The model under review builds one solid part; all positions refer to its coordinate system, in mm. A direction names the side the tool comes from. Coordinates: 2 decimals unless noted, no trailing zeros. Write each loop counter-clockwise with the first axis right and the second up, starting at its lowest first coordinate (ties: lowest second). Pieces come first, ordered by that corner, then holes. Notation, with made-up numbers: (50.25, 71.5) - (81.25, 71.5) arc R19 cw to (81.25, 87.5) - close; hole circle Ø7 at (-18.5, 46.25). An arc over 180 degrees is marked (long way). Put each result on its own line as item: value.
from build123d import *

# Parameters (mm, degrees)
SZKIC1_R                    = 1.5
DODANIE_WYCI_GNI_CIE1_DEPTH = 2
SZKIC2_W                    = 3
SZKIC2_H                    = 6
DODANIE_WYCI_GNI_CIE2_DEPTH = 10
SZKIC3_R                    = 1.5
WYTNIJ_WYCI_GNI_CIE1_DEPTH  = 3
SFAZOWANIE1_SIZE            = 1
SFAZOWANIE2_SIZE            = 1


with BuildPart() as part:
    # Szkic1 → Dodanie-wyciągnięcie1 (new body)
    with BuildSketch(Plane.XY):
        with BuildLine():
            Line((-6.716548808, 4.5), (7.283451192, 4.5))
            Line((7.283451192, 4.5), (7.283451192, 10.768070335))
            ThreePointArc((7.283451192, 10.768070335), (0.336426694, 12.995646082), (-6.716548808, 11.130497388))
            Line((-6.716548808, 11.130497388), (-6.716548808, 4.5))
        make_face()
        with Locations((0.283451192, 10.49617337)):
            Circle(SZKIC1_R, mode=Mode.SUBTRACT)
    extrude(amount=DODANIE_WYCI_GNI_CIE1_DEPTH)

    # Szkic2 → Dodanie-wyciągnięcie2 (add)
    with BuildSketch(Plane.XY.offset(2)):
        with Locations((5.783451192, 7.5)):
            Rectangle(SZKIC2_W, SZKIC2_H)
    extrude(amount=DODANIE_WYCI_GNI_CIE2_DEPTH)

    # Szkic3 → Wytnij-wyciągnięcie1 (cut)
    with BuildSketch(Plane.ZY.offset(-4.283451192)):
        with Locations((9, 7.579153313)):
            Circle(SZKIC3_R)
    extrude(amount=-WYTNIJ_WYCI_GNI_CIE1_DEPTH, mode=Mode.SUBTRACT)

    # Sfazowanie1
    sfazowanie1_edges = [part.edges().sort_by_distance(p)[0] for p in [
        (4.283451192, 7.5, 2),
    ]]
    chamfer(sfazowanie1_edges, length=SFAZOWANIE1_SIZE)

    # Sfazowanie2
    sfazowanie2_edges = [part.edges().sort_by_distance(p)[0] for p in [
        (5.283451192, 10.5, 2),
    ]]
    chamfer(sfazowanie2_edges, length=SFAZOWANIE2_SIZE)


solid = part.part
1. Consider section D-D on z = 5.5. State the section outline as (x, y) points.
Determined:
outline: (4.28, 4.5) - (7.28, 4.5) - (7.28, 10.5) - (4.28, 10.5) - close
2. To check wall thickness, follow probe 1 along X at (y, z) = (10.5, 0.5); probe 2 along X at (y, z) = (10.25, 6.25); probe 3 along Z at (x, y) = (-4.5, 10.25). State the ranges of each line that lie inside material, in increasing order.
Determined:
probe 1: x = -6.72 to -1.22, 1.78 to 7.28
probe 2: x = 4.28 to 7.28
probe 3: z = 0 to 2
3. Consider section B-B on y = 9.5. State the section outline as (x, z) points, plus the area to 3 significant figures.
Determined:
outline: (-6.72, 0) - (-0.84, 0) - (-0.84, 2) - (-6.72, 2) - close; (1.4, 0) - (7.28, 0) - (7.28, 12) - (4.28, 12) - (4.28, 3) - (3.28, 2) - (1.4, 2) - close
area: 54.0 mm^2
4. Consider section A-A on z = 9. State the section outline as (x, y) points.
Determined:
outline: (4.28, 4.5) - (7.28, 4.5) - (7.28, 6.08) - (4.28, 6.08) - close; (4.28, 9.08) - (7.28, 9.08) - (7.28, 10.5) - (4.28, 10.5) - close
5. For pin 1 Ø2 at (x, z) = (-5, 2) entering from +Y; pin 2 Ø4.5 at (x, y) = (0.5, 7) entering from +Z; pin 3 Ø0.9 at (x, z) = (5, 8.5) entering from +Y, all flat-tipped, find the tip position at first contact; note any pin that passes through.
Determined:
pin 1: stops at y = 12.37
pin 2: stops at z = 2
pin 3: stops at y = 10.5
6. Machinability: for faces 1 (the flat face through (-6.717, 8, 1)), 2 (the flat face through (6, 10.5, 7)), 3 (the flat face through (4.283, 7, 7)), which of the approach directions +Z, -Z, +X, -X, +Y, -Y give a long, thin tool a straight path to every point of the face, cutting with its end or side? Answer none if there is none.
Determined:
face 1: +Z, -Z, -X, +Y, -Y
face 2: +Z, +X, -X, +Y
face 3: +Z, -X, +Y, -Y
7. Consider section C-C on y = 7. State the section outline as (x, z) points.
Determined:
outline: (-6.72, 0) - (7.28, 0) - (7.28, 7.62) - (4.28, 7.62) - (4.28, 3) - (3.28, 2) - (-6.72, 2) - close; (4.28, 10.38) - (7.28, 10.38) - (7.28, 12) - (4.28, 12) - close
8. The part is to be moulded in two halves that separate along X. For faces 4 (the cylindrical face through (5.762, 6.666, 7.81)), 5 (the flat face through (7.283, 8, 6)), 6 (the flat face through (3.776, 7.951, 2.493)), 7 (the cylindrical face through (-0.04, 9.03, 0.99)), say which applies: +X half, -X half, draft (parallel to the pull), parting line (faces both ways), or undercut.
Determined:
face 4: draft
face 5: +X half
face 6: -X half
face 7: undercut
